Work out the finished part from the listing and answer in its coordinate system (mm). Round coordinates to 2 decimals unless told otherwise and drop trailing zeros. Order: outer loops, then holes, each group sorted by start corner. A loop starts at its lowest first (then second) coordinate and runs counter-clockwise, first axis right, second up. Notation, with made-up numbers: (58, -14) - (99, -14) arc R19 cw to (99, 16) - close; hole circle Ø6 at (-12.75, 22.5). An arc over 180 degrees is marked (long way). Put each result on its own line as item: value.
```python
from build123d import *

# Parameters (mm, degrees)
DODANIE_WYCI_GNI_CIE1_DEPTH = 10
WYTNIJ_WYCI_GNI_CIE1_REACH  = 98.949
SZKIC2_R                    = 9.99307311


with BuildPart() as part:
    # Szkic1 → Dodanie-wyciągnięcie1 (new body)
    with BuildSketch(Plane(origin=(0, 0, 0), x_dir=(1, 0, 0), z_dir=(0, 1, 0))):
        with BuildLine():
            Line((0, 30.032086689), (61.604280389, 30.032086689))
            ThreePointArc((61.604280389, 30.032086689), (91.636367078, 0), (61.604280389, -30.032086689))
            Line((61.604280389, -30.032086689), (0, -30.032086689))
            ThreePointArc((0, -30.032086689), (-30.032086689, 0), (0, 30.032086689))
        make_face()
    extrude(amount=DODANIE_WYCI_GNI_CIE1_DEPTH)

    # Szkic2 → Wytnij-wyciągnięcie1 (cut, up to next)
    with BuildSketch(Plane(origin=(0, 10, 0), x_dir=(1, 0, 0), z_dir=(0, 1, 0)), mode=Mode.PRIVATE) as wytnij_wyci_gni_cie1_sk1:
        with Locations(Location((0, 0, 0), (0, 0, 270))):
            Circle(SZKIC2_R)
    wytnij_wyci_gni_cie1_tool1 = extrude(wytnij_wyci_gni_cie1_sk1.sketch, amount=-WYTNIJ_WYCI_GNI_CIE1_REACH, mode=Mode.PRIVATE) & part.part
    add(wytnij_wyci_gni_cie1_tool1.solids().sort_by_distance((0, 10, 0))[0], mode=Mode.SUBTRACT)


solid = part.part
```
1) A cutting plane is placed at D-D on z = -25.5. Write down the section's boundary in (x, y).
Findings below:
outline: (-15.86, 0) - (77.47, 0) - (77.47, 10) - (-15.86, 10) - close
2) A cutting plane is placed at B-B on y = 2.5. Write down the section's boundary in (x, z).
Findings below:
outline: (0, -30.03) - (61.6, -30.03) arc R30.03 ccw to (61.6, 30.03) - (0, 30.03) arc R30.03 ccw to start; hole circle Ø19.99 at (0, 0)
3) Straight lines are drawn through the part: L1, parallel to X at y = 2.5, z = 0; L2, parallel to X at y = 3.5, z = 9; L3, parallel to X at y = 7.75, z = -25. For each, find the intervals that lie inside material, in ascending order. Write a range as from..to.
Findings below:
L1: x = -30.03..-9.99, 9.99..91.64
L2: x = -28.65..-4.34, 4.34..90.26
L3: x = -16.64..78.25
4) Given pin 1 Ø1 at (y, z) = (2, 18) entering from +X; pin 2 Ø6 at (x, y) = (78, 4) entering from +Z; pin 3 Ø3 at (x, y) = (-11, 2) entering from +Z, each flat-ended and moving along its own axis, determine where each tip first touches the part or whether it passes through.
Findings below:
pin 1: stops at x = 86.01
pin 2: stops at z = 26.88
pin 3: stops at z = 28.49
5) A cutting plane is placed at C-C on x = -21. Write down the section's boundary in (y, z), then the cut area to 3 significant figures.
Findings below:
outline: (0, -21.47) - (10, -21.47) - (10, 21.47) - (0, 21.47) - close
area: 429 mm2
6) For a pull along Z with two mould halves and no side action, classify faces 1 (the flat face through (32, 10, 0)), 2 (the cylindrical face through (0.439, 5.07, -9.983)), 3 (the flat face through (31, 5, 30.032)) as pulls with the +Z half, pulls with the -Z half, needs draft (parallel to the pull), parting line crosses it, or undercut.
Findings below:
face 1: needs draft
face 2: undercut
face 3: pulls with the +Z half
7) A cutting plane is placed at A-A on z = 0. Write down the section's boundary in (x, y).
Findings below:
outline: (-30.03, 0) - (-9.99, 0) - (-9.99, 10) - (-30.03, 10) - close; (9.99, 0) - (91.64, 0) - (91.64, 10) - (9.99, 10) - close
